from build123d import *

# Parameters (mm, degrees)
SKETCH_1_W          = 42
SKETCH_1_H          = 42
EXTRUDE_1_DEPTH     = 1.5
SKETCH_2_R          = 1.15
CUT_EXTRUDE_1_DEPTH = 2
SKETCH_3_R          = 8
EXTRUDE_2_DEPTH     = 24.9
SKETCH_4_W          = 16
SKETCH_4_H          = 16
EXTRUDE_3_DEPTH     = 7.4
SKETCH_5_R          = 8.75
EXTRUDE_4_DEPTH     = 3


with BuildPart() as part:
    # 草图1 → 凸台-拉伸1 (new body)
    with BuildSketch(Plane(origin=(0, 0, 0), x_dir=(1, 0, 0), z_dir=(0, 1, 0))):
        Rectangle(SKETCH_1_W, SKETCH_1_H)
    extrude(amount=EXTRUDE_1_DEPTH)

    # 草图2 → 切除-拉伸1 (cut)
    with BuildSketch(Plane(origin=(0, 1.5, 0), x_dir=(1, 0, 0), z_dir=(0, 1, 0))):
        with Locations(Location((-17, 17, 0), (0, 0, 270))):
            Circle(SKETCH_2_R)
        with Locations(Location((17, 17, 0), (0, 0, 270))):
            Circle(SKETCH_2_R)
        with Locations(Location((-17, -17, 0), (0, 0, 270))):
            Circle(SKETCH_2_R)
        with Locations(Location((17, -17, 0), (0, 0, 270))):
            Circle(SKETCH_2_R)
    extrude(amount=-CUT_EXTRUDE_1_DEPTH, mode=Mode.SUBTRACT)

    # 草图3 → 凸台-拉伸2 (add)
    with BuildSketch(Plane(origin=(0, 1.5, 0), x_dir=(1, 0, 0), z_dir=(0, 1, 0))):
        with Locations(Location((0, 0, 0), (0, 0, 270))):
            Circle(SKETCH_3_R)
    extrude(amount=EXTRUDE_2_DEPTH)

    # 草图4 → 凸台-拉伸3 (add)
    with BuildSketch(Plane(origin=(0, 1.5, 0), x_dir=(1, 0, 0), z_dir=(0, 1, 0))):
        Rectangle(SKETCH_4_W, SKETCH_4_H)
    extrude(amount=EXTRUDE_3_DEPTH)

    # 草图5 → 凸台-拉伸4 (add)
    with BuildSketch(Plane(origin=(0, 26.4, 0), x_dir=(1, 0, 0), z_dir=(0, 1, 0))):
        with Locations(Location((0, 0, 0), (0, 0, 270))):
            Circle(SKETCH_5_R)
    extrude(amount=EXTRUDE_4_DEPTH)


solid = part.part
Geometry check sheet. Reference: the model listing, model coordinates, mm. A direction names the side the tool comes from. Round coordinates to 2 decimals unless told otherwise and drop trailing zeros. Write each loop counter-clockwise with the first axis right and the second up, starting at its lowest first coordinate (ties: lowest second). Pieces come first, ordered by that corner, then holes. Notation, with made-up numbers: (74, 89.25) -> (107, 89.25) arc R9 ccw to (107, 94.25) -> close; hole circle Ø5 at (33, 84). An arc over 180 degrees is marked (long way). One line per item, written item: value. Start each with the question number.
(1) Cross-section at C-C, the plane z = 4. Record the cut outline in (x, y).
(2) Go/stop test with flat-tipped pins: pin 1 Ø2 at (y, z) = (4, -2) entering from -X; pin 2 Ø12 at (y, z) = (15.5, 9.5) entering from -X; pin 3 Ø2.5 at (x, z) = (17, 17) entering from +Y. Record where each tip stops, or that it passes through.
(3) Cross-section at B-B, the plane x = 17. Record the cut outline in (y, z).
(4) Scan lines: line 1 (X direction, y = 0.65, z = -17); line 2 (Y direction, x = -3, z = -15); line 3 (X direction, y = 19.75, z = 2). Record each from-to range of solid material in increasing order. Write a range as [from, to].
(5) Draft check along X on faces 6 (the flat face through (6, 8.9, -6)), 7 (the flat face through (8, 5, 0)), 8 (the cylindrical face through (-16.95, 0.76, -18.15)). Enter one of: +X half, -X half, draft (parallel to the pull), parting line (faces both ways), or undercut.
(6) Cross-section at D-D, the plane x = -10. Record the cut outline in (y, z).
(7) Cross-section at A-A, the plane z = -17. Record the cut outline in (x, y), and give its area (3 significant figures).
(8) Access from +Z, -Z, +X, -X, +Y, -Y to the whole of each face (thin tool, end or side, straight path). Record for faces 1 (the flat face through (-8, 5, 0)), 2 (the flat face through (-6, 8.9, -6)), 3 (the cylindrical face through (-5.324, 27.879, -6.944)), 4 (the cylindrical face through (-7.81, 17.53, -1.73)), 5 (the flat face through (0, 5, 8)).
Answer:
1. outline: (-21, 0) -> (21, 0) -> (21, 1.5) -> (8, 1.5) -> (8, 8.9) -> (6.93, 8.9) -> (6.93, 26.4) -> (7.78, 26.4) -> (7.78, 29.4) -> (-7.78, 29.4) -> (-7.78, 26.4) -> (-6.93, 26.4) -> (-6.93, 8.9) -> (-8, 8.9) -> (-8, 1.5) -> (-21, 1.5) -> close
2. pin 1: x = -8
2. pin 2: x = -7.19
2. pin 3: y = 1.5
3. outline: (0, -21) -> (1.5, -21) -> (1.5, -18.15) -> (0, -18.15) -> close; (0, -15.85) -> (1.5, -15.85) -> (1.5, 15.85) -> (0, 15.85) -> close; (0, 18.15) -> (1.5, 18.15) -> (1.5, 21) -> (0, 21) -> close
4. line 1: [-21, -18.15], [-15.85, 15.85], [18.15, 21]
4. line 2: [0, 1.5]
4. line 3: [-7.75, 7.75]
5. face 6: draft
5. face 7: +X half
5. face 8: undercut
6. outline: (0, -21) -> (1.5, -21) -> (1.5, 21) -> (0, 21) -> close
7. outline: (-21, 0) -> (-18.15, 0) -> (-18.15, 1.5) -> (-21, 1.5) -> close; (-15.85, 0) -> (15.85, 0) -> (15.85, 1.5) -> (-15.85, 1.5) -> close; (18.15, 0) -> (21, 0) -> (21, 1.5) -> (18.15, 1.5) -> close
7. area: 56.1 mm²
8. face 1: +Z, -Z, -X
8. face 2: -Z, -X
8. face 3: +Y
8. face 4: none
8. face 5: +Z, +X, -X
